Design review of the part built by this model. Coordinates are the model's own, in mm. A direction names the side the tool comes from. Round coordinates to 2 decimals unless told otherwise and drop trailing zeros. Write each loop counter-clockwise with the first axis right and the second up, starting at its lowest first coordinate (ties: lowest second). Pieces come first, ordered by that corner, then holes. Notation, with made-up numbers: (-22, 36) -> (23, 36) arc R29 cw to (23, 65) -> close; hole circle Ø5 at (49.25, 41). An arc over 180 degrees is marked (long way). One line per question, with ' | ' between items. Start each with the question number.
1) For faces 1 (the flat face through (0, 6.35, -73)), 2 (the flat face through (0, 3, 31.75)), 3 (the cylindrical face through (28.619, 36.808, -40.944)), list the 3-axis set-ups (+Z, -Z, +X, -X, +Y, -Y) from which the entire face can be reached by the end or side of a thin tool; tool diameter is ignored.
2) For probe 1 along X at (y, z) = (38, 52.5); probe 2 along Z at (x, y) = (13.5, 42); probe 3 along Z at (x, y) = (19.5, 9.5), list the stretches that pass through material, from the lowest coordinate up.
3) Consider section C-C (x = -5). Give the boundary of the cut face in (y, z), then the cut area to 3 significant figures.
4) Insertion check: pin 1 Ø6 at (y, z) = (12.065, 41.275) entering from +X; pin 2 Ø5 at (x, z) = (-7.5, -73) entering from +Y. Each pin has a flat end and moves straight along its axis. Give the tip position at first contact, or say it passes through.
5) Consider section A-A (z = 0). Give the boundary of the cut face in (x, y) (3 decimals).
6) Consider section B-B (y = 16.5). Give the boundary of the cut face in (x, z).
7) Mouldability with a two-part tool opening along Y and no side actions: class faces 4 (the flat face through (0, 25, 76.2)), 5 (the cylindrical face through (-28.531, 14.583, -40.944)), 6 (the cylindrical face through (-28.531, 36.808, -40.944)), 7 (the flat face through (0, 6.35, 73)) as +Y half, -Y half, draft (parallel to the pull), parting line (faces both ways), or undercut.
8) Consider section D-D (y = 34.29). Count the separate pieces of the cut face and the enclosed holes in it, then the cut area to 3 significant figures.
```python
from build123d import *

# Parameters (mm, degrees)
SKETCH1_W           = 50.8
SKETCH1_H           = 38.1
MOUNT_BASE_DEPTH    = 6.35
SKETCH5_W           = 63.5
SKETCH5_H           = 165.1
BOSS_EXTRUDE2_DEPTH = 38.1
SKETCH4_R           = 2.54
CUT_EXTRUDE1_DEPTH  = 114.236721076
OUTSIDE_VERTICES_R  = 12.7


with BuildPart() as part:
    # Sketch1 → Mount Base (new body)
    with BuildSketch(Plane(origin=(0, 0, 0), x_dir=(1, 0, 0), z_dir=(0, 1, 0))):
        Polygon((-31.75, 82.55), (-31.75, -82.55), (31.75, -82.55), (31.75, 82.55), (25.4, 82.55), align=None)
        with Locations((0, -50.8)):
            Rectangle(SKETCH1_W, SKETCH1_H, mode=Mode.SUBTRACT)
        Rectangle(SKETCH1_W, SKETCH1_H, mode=Mode.SUBTRACT)
        with Locations((0, 50.8)):
            Rectangle(SKETCH1_W, SKETCH1_H, mode=Mode.SUBTRACT)
    extrude(amount=MOUNT_BASE_DEPTH)

    # Sketch5 → Boss-Extrude2 (add)
    with BuildSketch(Plane(origin=(0, 6.35, 0), x_dir=(-1, 0, 0), z_dir=(0, 1, 0))):
        Rectangle(SKETCH5_W, SKETCH5_H)
        Polygon((25.4, -76.2), (-25.4, -76.2), (-25.4, -69.85), (-25.4, -31.75), (-25.4, -19.05), (-25.4, 19.05), (-25.4, 31.75), (-25.4, 69.85), (-25.4, 76.2), (25.4, 76.2), (25.4, 69.85), (25.4, 31.75), (25.4, 19.05), (25.4, -19.05), (25.4, -31.75), (25.4, -69.85), align=None, mode=Mode.SUBTRACT)
    extrude(amount=BOSS_EXTRUDE2_DEPTH)

    # Sketch4 → Cut-Extrude1 (cut, through all)
    with BuildSketch(Plane(origin=(31.75, 0, 0), x_dir=(0, 0, -1), z_dir=(1, 0, 0))):
        with Locations((0, 34.29)):
            Circle(SKETCH4_R)
        with Locations((41.275, 34.29)):
            Circle(SKETCH4_R)
        with Locations((-41.275, 34.29)):
            Circle(SKETCH4_R)
        with Locations((-41.275, 12.065)):
            Circle(SKETCH4_R)
        with Locations((41.275, 12.065)):
            Circle(SKETCH4_R)
        with Locations((0, 12.065)):
            Circle(SKETCH4_R)
    extrude(amount=-CUT_EXTRUDE1_DEPTH, mode=Mode.SUBTRACT)

    # Outside Vertices
    outside_vertices_edges = [part.edges().sort_by_distance(p)[0] for p in [
        (31.75, 22.225, 82.55),
        (-31.75, 22.225, 82.55),
        (-31.75, 22.225, -82.55),
        (31.75, 22.225, -82.55),
    ]]
    fillet(outside_vertices_edges, radius=OUTSIDE_VERTICES_R)


solid = part.part
```
From the geometry:
1) face 1: +Y | face 2: +Y, -Y | face 3: +X, -X
2) probe 1: x = -31.75 to -25.4, 25.4 to 31.75 | probe 2: z = -82.55 to -76.2, 76.2 to 82.55 | probe 3: z = -82.54 to -76.2, 76.2 to 82.54
3) outline: (0, -82.55) -> (44.45, -82.55) -> (44.45, -76.2) -> (6.35, -76.2) -> (6.35, -69.85) -> (0, -69.85) -> close; (0, -31.75) -> (6.35, -31.75) -> (6.35, -19.05) -> (0, -19.05) -> close; (0, 19.05) -> (6.35, 19.05) -> (6.35, 31.75) -> (0, 31.75) -> close; (0, 69.85) -> (6.35, 69.85) -> (6.35, 76.2) -> (44.45, 76.2) -> (44.45, 82.55) -> (0, 82.55) -> close | area: 806 mm2
4) pin 1: stops at x = 31.75 | pin 2: stops at y = 6.35
5) outline: (-31.75, 0) -> (-25.4, 0) -> (-25.4, 9.525) -> (-31.75, 9.525) -> close; (-31.75, 14.605) -> (-25.4, 14.605) -> (-25.4, 31.75) -> (-31.75, 31.75) -> close; (-31.75, 36.83) -> (-25.4, 36.83) -> (-25.4, 44.45) -> (-31.75, 44.45) -> close; (25.4, 0) -> (31.75, 0) -> (31.75, 9.525) -> (25.4, 9.525) -> close; (25.4, 14.605) -> (31.75, 14.605) -> (31.75, 31.75) -> (25.4, 31.75) -> close; (25.4, 36.83) -> (31.75, 36.83) -> (31.75, 44.45) -> (25.4, 44.45) -> close
6) outline: (-31.75, -69.85) arc R12.7 ccw to (-19.05, -82.55) -> (19.05, -82.55) arc R12.7 ccw to (31.75, -69.85) -> (31.75, 69.85) arc R12.7 ccw to (19.05, 82.55) -> (-19.05, 82.55) arc R12.7 ccw to (-31.75, 69.85) -> close; hole (-25.4, -76.2) -> (25.4, -76.2) -> (25.4, 76.2) -> (-25.4, 76.2) -> close
7) face 4: draft | face 5: undercut | face 6: undercut | face 7: +Y half
8) separate pieces: 6 | enclosed holes: 0 | area: 2,410 mm2
